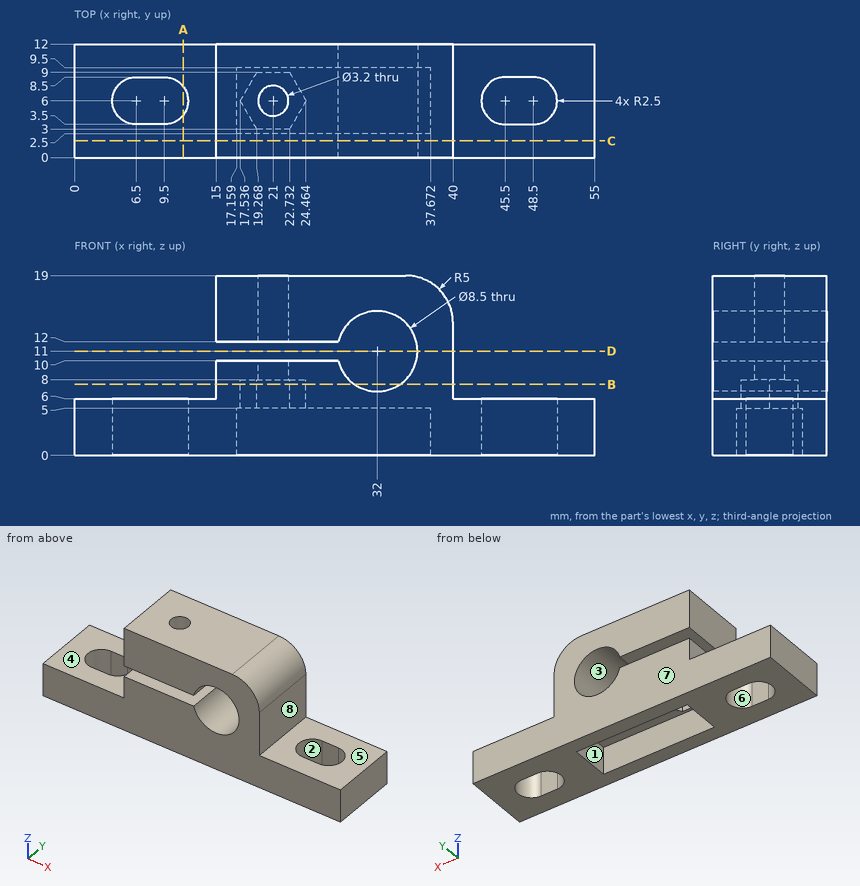
Print and shaded views of the part. All mm, measured from the part's lowest x, y and z. A direction names the side the tool comes from. Round coordinates to 2 decimals unless told otherwise and drop trailing zeros. Write each loop counter-clockwise with the first axis right and the second up, starting at its lowest first coordinate (ties: lowest second). Pieces come first, ordered by that corner, then holes.
Item 1: Two-plate mould, pull along Y, no slides. Class the marked faces 6, 7 and 8: +Y half, -Y half, draft (parallel to the pull), parting line (faces both ways), or undercut.
Results:
face 6: undercut
face 7: +Y half
face 8: draft
Item 2: Cut at A-A, the plane x = 11.5. Give the cut face in (y, z).
Results:
outline: (0, 0) - (4.5, 0) - (4.5, 6) - (0, 6) - close; (7.5, 0) - (12, 0) - (12, 6) - (7.5, 6) - close
Item 3: Probe L1, parallel to Y at x = 26, z = 3.5; L2, parallel to Y at x = 21, z = 9.25; L3, parallel to X at y = 4.5, z = 1. List the from-to ranges inside material, lowest first.
Results:
L1: y = 0 to 2.5, 9.5 to 12
L2: y = 0 to 4.4, 7.6 to 12
L3: x = 0 to 4.5, 11.5 to 17.16, 37.67 to 43.5, 50.5 to 55
Item 4: Cut at D-D, the plane z = 11. Give the cut face in (x, y).
Results:
outline: (36.25, 0) - (40, 0) - (40, 12) - (36.25, 12) - close
Item 5: Cut at B-B, the plane z = 7.5. Give the cut face in (x, y) (1 decimal), plus the area to 3 significant figures.
Results:
outline: (15, 0) - (29.6, 0) - (29.6, 12) - (15, 12) - close; (34.4, 0) - (40, 0) - (40, 12) - (34.4, 12) - close; hole (17.5, 6) - (19.3, 3) - (22.7, 3) - (24.5, 6) - (22.7, 9) - (19.3, 9) - close
area: 211 mm2
Item 6: Drop flat-ended pins along their axis: pin 1 Ø3.5 at (x, y) = (6, 8) entering from +Z; pin 2 Ø5.5 at (x, z) = (32.5, 2.5) entering from -Y; pin 3 Ø2 at (y, z) = (5.5, 17) entering from -X; pin 4 Ø6 at (y, z) = (4, 15) entering from +X. Give the stop position or say it passes through.
Results:
pin 1: stops at z = 6
pin 2: stops at y = 0
pin 3: stops at x = 15
pin 4: stops at x = 40
Item 7: Cut at C-C, the plane y = 1.75. Give the cut face in (x, z).
Results:
outline: (0, 0) - (55, 0) - (55, 6) - (40, 6) - (40, 14) arc R5 ccw to (35, 19) - (15, 19) - (15, 12) - (27.87, 12) arc R4.25 cw (long way) to (27.87, 10) - (15, 10) - (15, 6) - (0, 6) - close
Item 8: Which spindle directions (+Z, -Z, +X, -X, +Y, -Y) get a long thin tool onto all of the face, cutting with end or side? Do the marked faces 1, 2, 3, 4 and 5. Say none if no direction does.
Results:
face 1: -Z
face 2: +Z, -Z
face 3: +Y, -Y
face 4: +Z, -X, +Y, -Y
face 5: +Z, +X, +Y, -Y
